Source: CAD feature listing. Evaluate the final solid. Frame: model axes, mm. A direction names the side the tool comes from. Give positions to 0.01 mm unless a question says otherwise; leave off trailing zeros. Order: outer loops, then holes, each group sorted by start corner. A loop starts at its lowest first (then second) coordinate and runs counter-clockwise, first axis right, second up. Notation, with made-up numbers: M -18.75,-27.75 L 34.25,-27.75 A21 ccw 34.25,8.25 Z; hole C 39,13.25 d5. An arc over 180 degrees is marked long. Answer as a JSON object with one key per item and string values. Group by question number.
1. Material intervals for L1, parallel to Y at x = 11, z = 2.9; L2, parallel to Y at x = 12, z = 3.25; L3, parallel to X at y = 24, z = 4.7, sorted ascending. Write a range as [from, to].
2. Section query B-B (z = 4.05). Output: boundary loops of the cut face in (x, y), plus the area to 3 significant figures.
3. Set-up query: faces 1 (the cylindrical face through (19.5, 6.7, 2.5)), 2 (the flat face through (0, 26, 2)), 3 (the conical face through (19.62, 45.1, 0.13)), 4 (the conical face through (2.38, 6.9, 4.87)), 5 (the flat face through (18, 32, 5)). Return all of +Z, -Z, +X, -X, +Y, -Y with unobstructed straight access to the full face (end or side cutting, diameter ignored); none if empty.
4. Section query C-C (y = 6.8). Output: boundary loops of the cut face in (x, z).
5. Pull-direction query (X, two-part tool) for faces 6 (the flat face through (22, 26, 2)), 7 (the flat face through (11, 0, 2)), 8 (the flat face through (11, 11.3, 3)), 9 (the cylindrical face through (2.5, 6.9, 2.5)); classes: +X half, -X half, draft (parallel to the pull), parting line (faces both ways), or undercut.
6. Section query A-A (y = 26). Output: boundary loops of the cut face in (x, z), plus the area to 4 significant figures.
7. Section query D-D (x = 4.5). Count the separate pieces of the cut face and the enclosed holes in it, plus the area to 3 significant figures.
from build123d import *

# Parameters (mm, degrees)
ESQUISSE1_W             = 22
ESQUISSE1_H             = 52
BOSS_EXTRU_1_DEPTH      = 5
ESQUISSE5_R             = 8
ENL_V_MAT_EXTRU_2_DEPTH = 5
ENL_V_MAT_EXTRU_3_DEPTH = 57.683330883
CHANFREIN1_SIZE         = 0.25


with BuildPart() as part:
    # Esquisse1 → Boss.-Extru.1 (new body)
    with BuildSketch(Plane.XY):
        with Locations((11, 26)):
            Rectangle(ESQUISSE1_W, ESQUISSE1_H)
    extrude(amount=BOSS_EXTRU_1_DEPTH)

    # Esquisse5 → Enlèv. mat.-Extru.2 (cut)
    with BuildSketch(Plane.XY.offset(5)):
        with Locations((11, 26)):
            Circle(ESQUISSE5_R)
    extrude(amount=-ENL_V_MAT_EXTRU_2_DEPTH, mode=Mode.SUBTRACT)

    # Esquisse6 → Enlèv. mat.-Extru.3 (cut, through all)
    with BuildSketch(Plane.XY.offset(5)):
        with BuildLine():
            Line((7, 49.7), (15, 49.7))
            ThreePointArc((15, 49.7), (19.5, 45.2), (15, 40.7))
            Line((15, 40.7), (7, 40.7))
            ThreePointArc((7, 40.7), (2.5, 45.2), (7, 49.7))
        make_face()
        with BuildLine():
            Line((7, 2.3), (15, 2.3))
            ThreePointArc((15, 2.3), (19.5, 6.8), (15, 11.3))
            Line((15, 11.3), (7, 11.3))
            ThreePointArc((7, 11.3), (2.5, 6.8), (7, 2.3))
        make_face()
    extrude(amount=-ENL_V_MAT_EXTRU_3_DEPTH, mode=Mode.SUBTRACT)

    # Chanfrein1
    chanfrein1_edges = [part.edges().sort_by_distance(p)[0] for p in [
        (22, 26, 5),
        (11, 52, 5),
        (3, 26, 0),
        (3, 26, 5),
        (2.5, 45.2, 0),
        (11, 49.7, 0),
        (19.5, 45.2, 0),
        (11, 40.7, 0),
        (2.5, 45.2, 5),
        (11, 40.7, 5),
        (19.5, 45.2, 5),
        (11, 49.7, 5),
        (2.5, 6.8, 0),
        (11, 11.3, 0),
        (19.5, 6.8, 0),
        (11, 2.3, 0),
        (2.5, 6.8, 5),
        (11, 2.3, 5),
        (19.5, 6.8, 5),
        (11, 11.3, 5),
        (0, 26, 5),
        (11, 52, 0),
        (22, 26, 0),
        (11, 0, 0),
        (0, 26, 0),
        (11, 0, 5),
        (0, 52, 2.5),
        (22, 52, 2.5),
        (22, 0, 2.5),
        (0, 0, 2.5),
    ]]
    chamfer(chanfrein1_edges, length=CHANFREIN1_SIZE)


solid = part.part
Answer sheet:
{
 "1": {"L1": "[0, 2.3], [11.3, 18], [34, 40.7], [49.7, 52]", "L2": "[0, 2.3], [11.3, 18.06], [33.94, 40.7], [49.7, 52]", "L3": "[0, 3.25], [18.75, 22]"},
 "2": {"outline": "M 0,0.25 L 0.25,0 L 21.75,0 L 22,0.25 L 22,51.75 L 21.75,52 L 0.25,52 L 0,51.75 Z; hole C 11,26 d16; hole M 7,2.3 L 15,2.3 A4.5 ccw 15,11.3 L 7,11.3 A4.5 ccw Z; hole M 7,40.7 L 15,40.7 A4.5 ccw 15,49.7 L 7,49.7 A4.5 ccw Z", "area": "672 mm^2"},
 "3": {"face 1": "+Z, -Z", "face 2": "+Z, -Z, -X, +Y, -Y", "face 3": "-Z", "face 4": "+Z", "face 5": "+Z, +X, -X, +Y, -Y"},
 "4": {"outline": "M 0,0.25 L 0.25,0 L 2.25,0 L 2.5,0.25 L 2.5,4.75 L 2.25,5 L 0.25,5 L 0,4.75 Z; M 19.5,0.25 L 19.75,0 L 21.75,0 L 22,0.25 L 22,4.75 L 21.75,5 L 19.75,5 L 19.5,4.75 Z"},
 "5": {"face 6": "+X half", "face 7": "draft", "face 8": "undercut", "face 9": "undercut"},
 "6": {"outline": "M 0,0.25 L 0.25,0 L 2.75,0 L 3,0.25 L 3,4.75 L 2.75,5 L 0.25,5 L 0,4.75 Z; M 19,0.25 L 19.25,0 L 21.75,0 L 22,0.25 L 22,4.75 L 21.75,5 L 19.25,5 L 19,4.75 Z", "area": "29.75 mm^2"},
 "7": {"separate pieces": "4", "enclosed holes": "0", "area": "138 mm^2"}
}
